Autodesk Inventor part; units mm, degrees
ref_plane "YZ Plane" through (0, 0, 0) normal (1, 0, 0) x (0, 1, 0)
ref_plane "XZ Plane" through (0, 0, 0) normal (0, 1, 0) x (-1, 0, 0)
ref_plane "XY Plane" through (0, 0, 0) normal (0, 0, 1) x (1, 0, 0)
sketch "Sketch1" plane through (0, 0, 0) normal (0, 1, 0) x (-1, 0, 0)
  circle A0 centre (0, 0) radius 21
  dimension "d0" = 42
extrude "Extrusion1" add sketch "Sketch1" along normal blind 1
sketch "Sketch2" plane through (0, 1, 0) normal (0, 1, 0) x (1, 0, 0)
  circle A0 centre (0, 0) radius 16
  dimension "d3" = 32
extrude "Extrusion2" add sketch "Sketch2" along normal blind 7
sketch "Sketch3" plane through (0, 8, 0) normal (0, 1, 0) x (1, 0, 0)
  circle A0 centre (0, 0) radius 21
extrude "Extrusion3" add sketch "Sketch3" along normal blind 1
sketch "Sketch4" plane through (0, 9, 0) normal (0, 1, 0) x (1, 0, 0)
  circle A0 centre (0, 0) radius 12.5
  dimension "d8" = 25
extrude "Extrusion4" add sketch "Sketch4" along normal blind 7
sketch "Sketch5" plane through (0, 16, 0) normal (0, 1, 0) x (1, 0, 0)
  circle A0 centre (0, 0) radius 2.5
  dimension "d11" = 5
extrude "Extrusion5" cut sketch "Sketch5" against normal through all
properties part number "GT2 60T"
Source: CAD feature listing. Evaluate the final solid. Frame: model axes, mm. A direction names the side the tool comes from. Coordinates: 2 decimals unless noted, no trailing zeros. Order: outer loops, then holes, each group sorted by start corner. A loop starts at its lowest first (then second) coordinate and runs counter-clockwise, first axis right, second up.
Item 1: Cut plane D-D (x = -6). Return loops of the section in (y, z), plus the area to 3 significant figures.
Output values:
outline: (0, -20.12) - (1, -20.12) - (1, -14.83) - (8, -14.83) - (8, -20.12) - (9, -20.12) - (9, -10.97) - (16, -10.97) - (16, 10.97) - (9, 10.97) - (9, 20.12) - (8, 20.12) - (8, 14.83) - (1, 14.83) - (1, 20.12) - (0, 20.12) - close
area: 442 mm2
Item 2: Set-up query: faces 1 (the face through (4.8, 1, -15.5)), 2 (the face through (20.03, 8.49, 6.31)), 3 (the face through (9, 9, 9)). Return all of +Z, -Z, +X, -X, +Y, -Y with unobstructed straight access to the full face (end or side cutting, diameter ignored); none if empty.
Output values:
face 1: none
face 2: +Y, -Y
face 3: +Y
Item 3: Material intervals for line 1 (Z direction, x = 0, y = 8.5); line 2 (Y direction, x = 14, z = -14.5); line 3 (X direction, y = 5.5, z = 0), sorted ascending.
Output values:
line 1: z = -21 to -2.5, 2.5 to 21
line 2: y = 0 to 1, 8 to 9
line 3: x = -16 to -2.5, 2.5 to 16
Item 4: Cut plane A-A (x = 0). Return loops of the section in (y, z), plus the area to 3 significant figures.
Output values:
outline: (0, -21) - (1, -21) - (1, -16) - (8, -16) - (8, -21) - (9, -21) - (9, -12.5) - (16, -12.5) - (16, -2.5) - (0, -2.5) - close; (0, 2.5) - (16, 2.5) - (16, 12.5) - (9, 12.5) - (9, 21) - (8, 21) - (8, 16) - (1, 16) - (1, 21) - (0, 21) - close
area: 403 mm2
Item 5: First-contact query: P1, Ø4, axis at y = 4, z = 1, coming from the +X side; P2, Ø2, axis at x = 16, z = 7, coming from the +Y side; P3, Ø2, axis at x = -3.5, y = 9, coming from the -Z side. Flat tips, straight axial feed; report the tip coordinate or a pass-through.
Output values:
P1: stops at x = 16
P2: stops at y = 9
P3: stops at z = -20.85
Item 6: Cut plane B-B (z = 0). Return loops of the section in (x, y).
Output values:
outline: (-21, 0) - (-2.5, 0) - (-2.5, 16) - (-12.5, 16) - (-12.5, 9) - (-21, 9) - (-21, 8) - (-16, 8) - (-16, 1) - (-21, 1) - close; (2.5, 0) - (21, 0) - (21, 1) - (16, 1) - (16, 8) - (21, 8) - (21, 9) - (12.5, 9) - (12.5, 16) - (2.5, 16) - close
Item 7: Cut plane C-C (y = 1.75). Return loops of the section in (x, z).
Output values:
outline: circle Ø32 at (0, 0); hole circle Ø5 at (0, 0)
Item 8: Pull-direction query (Y, two-part tool) for faces 4 (the face through (-4.8, 8, 15.5)), 5 (the face through (-20.03, 0.49, -6.31)), 6 (the face through (-4, 0, 0)); classes: pulls with the +Y half, pulls with the -Y half, needs draft (parallel to the pull), parting line crosses it, or undercut.
Output values:
face 4: undercut
face 5: needs draft
face 6: pulls with the -Y half
